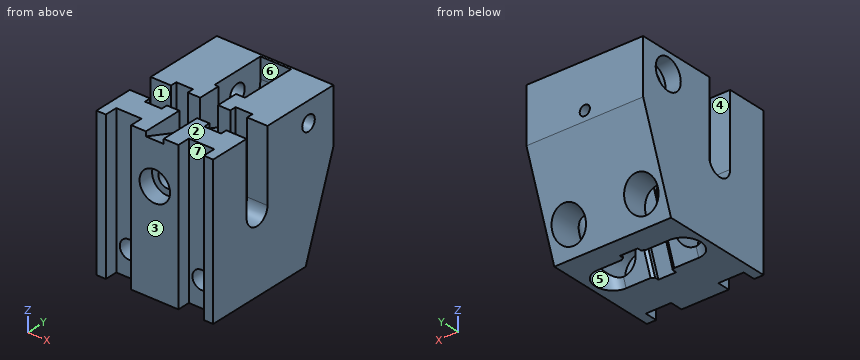
```python
from build123d import *

# Parameters (mm, degrees)
SKETCH1_W                = 23
SKETCH1_H                = 32.5
BOSS_EXTRUDE1_DEPTH      = 18
SKETCH2_W                = 23
SKETCH2_H                = 25
BOSS_EXTRUDE2_DEPTH      = 15
CHAMFER1_SIZE            = 15
SKETCH3_R                = 1.8
CUT_EXTRUDE1_DEPTH       = 44.694965385
CUT_EXTRUDE2_DEPTH       = 44.694965385
CUT_EXTRUDE3_START       = -4
CUT_EXTRUDE3_DEPTH       = 3.3
SKETCH7_W                = 5
SKETCH7_H                = 2.5
CUT_EXTRUDE4_DEPTH       = 52.713151132
CUT_EXTRUDE5_START       = -6.5
SKETCH8_R                = 3.25
CUT_EXTRUDE5_DEPTH       = 38.194965385
SKETCH9_R                = 1
CUT_EXTRUDE6_DEPTH       = 8
CUT_EXTRUDE8_DEPTH       = 1.75
CUT_EXTRUDE7_DEPTH       = 1.75
CUT_EXTRUDE9_DEPTH       = 13
SKETCH15_R               = 1.35
CUT_EXTRUDE10_DEPTH      = 6
CUT_EXTRUDE11_DEPTH      = 2.5
CUT_EXTRUDE11_DEPTH_BACK = 3.5
SKETCH17_R               = 1.75
CUT_EXTRUDE12_DEPTH      = 9
SKETCH18_R               = 3
CUT_EXTRUDE13_DEPTH      = 3
SKETCH19_R               = 1.5
CUT_EXTRUDE14_DEPTH      = 44.694965459
SKETCH20_R               = 1.75
CUT_EXTRUDE15_DEPTH      = 8
SKETCH21_R               = 3
CUT_EXTRUDE16_DEPTH      = 3
SKETCH22_R               = 1.5
CUT_EXTRUDE17_DEPTH      = 17
CUT_EXTRUDE18_DEPTH      = 44.694965459


with BuildPart() as part:
    # Sketch1 → Boss-Extrude1 (new body)
    with BuildSketch(Plane.XY):
        with Locations((11.5, 16.25)):
            Rectangle(SKETCH1_W, SKETCH1_H)
    extrude(amount=BOSS_EXTRUDE1_DEPTH)

    # Sketch2 → Boss-Extrude2 (add)
    with BuildSketch(Plane(origin=(0, 0, 0), x_dir=(-1, 0, 0), z_dir=(0, 0, -1))):
        with Locations((-11.5, 12.5)):
            Rectangle(SKETCH2_W, SKETCH2_H)
    extrude(amount=BOSS_EXTRUDE2_DEPTH)

    # Chamfer1
    # the kernel refuses this chamfer: 15 mm, written as the material it adds along each edge
    with BuildSketch(Plane(origin=(23, 25, 0), x_dir=(0, -0.02749587661058632, -0.9996219169112968), z_dir=(-1, 0, 0))) as chamfer1_piece_1_section:
        Polygon((CHAMFER1_SIZE * 0.999621916911, -CHAMFER1_SIZE * 0.0274958766106), (-CHAMFER1_SIZE * 0.0274958766106, -CHAMFER1_SIZE * 0.999621916911), (0, 0), align=None)
    chamfer1_piece_1 = extrude(amount=23, mode=Mode.PRIVATE)
    chamfer1_piece_1 = split(chamfer1_piece_1, bisect_by=Plane(origin=(11.5, 28.131672391, -15), z_dir=(0, 0, 1)), keep=Keep.TOP, mode=Mode.PRIVATE)
    chamfer1_piece_1 = split(chamfer1_piece_1, bisect_by=Plane(origin=(11.5, 32.5, -5.879790556), z_dir=(0, -1, 0)), keep=Keep.TOP, mode=Mode.PRIVATE)
    add(chamfer1_piece_1)

    # Sketch3 → Cut-Extrude1 (cut, through all)
    with BuildSketch(Plane.XZ):
        with Locations(Location((4.35, -10, 0), (0, 0, 270))):
            Circle(SKETCH3_R)
        with Locations(Location((18.65, -10, 0), (0, 0, 270))):
            Circle(SKETCH3_R)
    extrude(amount=-CUT_EXTRUDE1_DEPTH, mode=Mode.SUBTRACT)

    # Sketch4 → Cut-Extrude2 (cut, through all)
    with BuildSketch(Plane.ZY):
        with BuildLine():
            Line((0, 13), (18, 13))
            Line((18, 13), (18, 8))
            Line((18, 8), (0, 8))
            ThreePointArc((0, 8), (-2.5, 10.5), (0, 13))
        make_face()
    extrude(amount=-CUT_EXTRUDE2_DEPTH, mode=Mode.SUBTRACT)

    # Sketch5 → Cut-Extrude3 (cut)
    with BuildSketch(Plane.ZY.offset(CUT_EXTRUDE3_START)):
        Polygon((2.165063509, 14.25), (-2.165063509, 14.25), (-4.330127019, 10.5), (-2.165063509, 6.75), (2.165063509, 6.75), (18, 6.75), (18, 14.25), align=None)
    cut_extrude3 = extrude(amount=-CUT_EXTRUDE3_DEPTH, mode=Mode.SUBTRACT)

    # Sketch7 → Cut-Extrude4 (cut, through all)
    with BuildSketch(Plane(origin=(0, 0, -15), x_dir=(-1, 0, 0), z_dir=(0, 0, -1))):
        with Locations((-4.35, 1.25)):
            Rectangle(SKETCH7_W, SKETCH7_H)
    cut_extrude4 = extrude(amount=-CUT_EXTRUDE4_DEPTH, mode=Mode.SUBTRACT)

    # Sketch8 → Cut-Extrude5 (cut, through all)
    with BuildSketch(Plane.XZ.offset(CUT_EXTRUDE5_START)):
        with Locations(Location((4.35, -10, 0), (0, 0, 270))):
            Circle(SKETCH8_R)
    cut_extrude5 = extrude(amount=-CUT_EXTRUDE5_DEPTH, mode=Mode.SUBTRACT)

    # Mirror1: Cut-Extrude3, Cut-Extrude4, Cut-Extrude5 across plane
    add(cut_extrude3.mirror(Plane.ZY.offset(-11.5)), mode=Mode.SUBTRACT)
    add(cut_extrude4.mirror(Plane.ZY.offset(-11.5)), mode=Mode.SUBTRACT)
    add(cut_extrude5.mirror(Plane.ZY.offset(-11.5)), mode=Mode.SUBTRACT)

    # Sketch9 → Cut-Extrude6 (cut)
    with BuildSketch(Plane(origin=(0, 32.5, 0), x_dir=(1, 0, 0), z_dir=(0, 1, 0))):
        with Locations(Location((11.5, -5.25, 0), (0, 0, 270))):
            Circle(SKETCH9_R)
    extrude(amount=-CUT_EXTRUDE6_DEPTH, mode=Mode.SUBTRACT)

    # Sketch10 → Cut-Extrude8 (cut, symmetric)
    with BuildSketch(Plane.ZY.offset(-11.5)):
        Polygon((4.25, 24.5), (18, -13.277814518), (31.330171166, -4.978014809), (56.797179747, 10.878576059), (6.25, 24.5), align=None)
    extrude(amount=CUT_EXTRUDE8_DEPTH, both=True, mode=Mode.SUBTRACT)

    # Sketch11 → Cut-Extrude7 (cut, symmetric)
    with BuildSketch(Plane.ZY.offset(-11.5)):
        Polygon((1.029605681, 24.137976813), (5.29394834, 23.386058148), (6.774939004, 19.317069741), (3.991587008, 16), (-15, 9.087627628), (-15, 18.303677479), align=None)
    extrude(amount=CUT_EXTRUDE7_DEPTH, both=True, mode=Mode.SUBTRACT)

    # Sketch12 → Cut-Revolve2 (revolve, cut)
    with BuildSketch(Plane.ZY.offset(-11.5)):
        Polygon((0.20282315, 23.485738747), (1.570903724, 19.726968263), (-16.480990664, 13.156616034), (-17.849071237, 16.915386518), align=None)
    revolve(axis=Axis((11.5, 19.726968263, 1.570903724), (0, -0.34202014332567215, -0.9396926207859072)), mode=Mode.SUBTRACT)

    # Sketch13 → Cut-Extrude9 (cut)
    with BuildSketch(Plane(origin=(0, -3.757856581, -10.324626103), x_dir=(1, 0, 0), z_dir=(0, 0.34202014332567177, 0.9396926207859073))):
        with BuildLine():
            Line((18.65, 21.250005791), (11.5, 21.250005791))
            Line((11.5, 21.250005791), (11.5, 14.750005791))
            Line((11.5, 14.750005791), (18.65, 14.750005791))
            ThreePointArc((18.65, 14.750005791), (21.9, 18.000005791), (18.65, 21.250005791))
        make_face()
    cut_extrude9 = extrude(amount=CUT_EXTRUDE9_DEPTH, mode=Mode.SUBTRACT)

    # Sketch15 → Cut-Extrude10 (cut)
    with BuildSketch(Plane(origin=(0, 0.688405282, 1.891377967), x_dir=(-1, 0, 0), z_dir=(0, -0.34202014332567177, -0.9396926207859073))):
        with Locations(Location((-18.65, 18.000005791, 0), (0, 0, 90))):
            Circle(SKETCH15_R)
    cut_extrude10 = extrude(amount=-CUT_EXTRUDE10_DEPTH, mode=Mode.SUBTRACT)

    # Mirror2: Cut-Extrude9, Cut-Extrude10 across plane
    add(cut_extrude9.mirror(Plane.ZY.offset(-11.5)), mode=Mode.SUBTRACT)
    add(cut_extrude10.mirror(Plane.ZY.offset(-11.5)), mode=Mode.SUBTRACT)

    # Sketch16 → Cut-Extrude11 (cut, two sides: drawn at the far end of the back side and taken through both)
    with BuildSketch(Plane.ZY.offset(-11.5).offset(-CUT_EXTRUDE11_DEPTH_BACK)):
        with BuildLine():
            Line((10.075121942, 28.322250561), (25.575121942, 28.322250561))
            Line((25.575121942, 28.322250561), (25.575121942, 17.322250561))
            Line((25.575121942, 17.322250561), (10.075121942, 17.322250561))
            ThreePointArc((10.075121942, 17.322250561), (4.575121942, 22.822250561), (10.075121942, 28.322250561))
        make_face()
    extrude(amount=CUT_EXTRUDE11_DEPTH + CUT_EXTRUDE11_DEPTH_BACK, mode=Mode.SUBTRACT)

    # Sketch17 → Cut-Extrude12 (cut)
    with BuildSketch(Plane.ZY):
        with Locations((10.075121942, 22.822250561)):
            Circle(SKETCH17_R)
    extrude(amount=-CUT_EXTRUDE12_DEPTH, mode=Mode.SUBTRACT)

    # Sketch18 → Cut-Extrude13 (cut)
    with BuildSketch(Plane.ZY):
        with Locations((10.075121942, 22.822250561)):
            Circle(SKETCH18_R)
    extrude(amount=-CUT_EXTRUDE13_DEPTH, mode=Mode.SUBTRACT)

    # Sketch19 → Cut-Extrude14 (cut, through all)
    with BuildSketch(Plane.ZY):
        with Locations((10.075121942, 22.822250561)):
            Circle(SKETCH19_R)
    extrude(amount=-CUT_EXTRUDE14_DEPTH, mode=Mode.SUBTRACT)

    # Sketch20 → Cut-Extrude15 (cut)
    with BuildSketch(Plane.XZ):
        with Locations(Location((11.5, 5, 0), (0, 0, 270))):
            Circle(SKETCH20_R)
    extrude(amount=-CUT_EXTRUDE15_DEPTH, mode=Mode.SUBTRACT)

    # Sketch21 → Cut-Extrude16 (cut)
    with BuildSketch(Plane.XZ):
        with Locations(Location((11.5, 5, 0), (0, 0, 270))):
            Circle(SKETCH21_R)
    extrude(amount=-CUT_EXTRUDE16_DEPTH, mode=Mode.SUBTRACT)

    # Sketch22 → Cut-Extrude17 (cut)
    with BuildSketch(Plane.XZ):
        with Locations(Location((11.5, 5, 0), (0, 0, 222.242919533))):
            Circle(SKETCH22_R)
    extrude(amount=-CUT_EXTRUDE17_DEPTH, mode=Mode.SUBTRACT)

    # Sketch23 → Cut-Extrude18 (cut, through all)
    with BuildSketch(Plane(origin=(0, 0, 0), x_dir=(0, 0, -1), z_dir=(1, 0, 0))):
        Polygon((-18, 32.5), (-14.075121942, 32.5), (-13.4247686, 32.5), (15, 32.5), (15, 22.154230314), (-3.320235061, 28.822250561), (-14.075121942, 28.822250561), (-14.075121942, 0), (-18, 0), align=None)
    extrude(amount=CUT_EXTRUDE18_DEPTH, mode=Mode.SUBTRACT)


solid = part.part
```
The model under review builds one solid part; all positions refer to its coordinate system, in mm. Face numbers are marked on the shaded views. A direction names the side the tool comes from. Round coordinates to 2 decimals unless told otherwise and drop trailing zeros. Loops run counter-clockwise (first coordinate to the right, second up) from the corner with the lowest first, then second, coordinate; pieces in that order, holes last. Notation, with made-up numbers: M 5,70.5 L 53,70.5 A22 cw 53,106.5 Z; hole C 62,58.25 d7. An arc over 180 degrees is marked long. Put each result on its own line as item: value.
Q1. Machinability: for the marked faces 4, 5, 6 and 7, which of the approach directions +Z, -Z, +X, -X, +Y, -Y give a long, thin tool a straight path to every point of the face, cutting with its end or side? Answer none if there is none.
Result set:
face 4: +Z, +X, -X
face 5: none
face 6: +Z
face 7: +Z, -Z, -Y
Q2. Consider section A-A, the plane y = 8.5. Give the boundary of the cut face in (x, z).
Result set:
outline: M 0,-15 L 23,-15 L 23,-1.5 L 19,-1.5 L 19,-3.18 L 15.7,-3.18 L 15.7,-1.5 L 7.3,-1.5 L 7.3,-3.18 L 4,-3.18 L 4,-1.5 L 0,-1.5 Z; hole C 4.35,-10 d6.5; hole C 18.65,-10 d6.5
Q3. To check wall thickness, follow L1, parallel to X at y = 7.05, z = 5; L2, parallel to X at y = 19.25, z = 11.5; L3, parallel to X at y = 16, z = 5. State the ranges of each line that lie inside material, in increasing order.
Result set:
L1: x = 0 to 4, 7.3 to 9.75, 13.25 to 15.7, 19 to 23
L2: x = 0 to 9, 15 to 23
L3: x = 0 to 10, 13 to 23
Q4. For pin 1 (5 mm diameter, centred on y = 19.5, z = 0.5, fed in from -X); pin 2 (12 mm diameter, centred on x = 6.5, z = -6.5, fed in from +Y); pin 3 (1.2 mm diameter, centred on x = 11.5, z = 5.25, fed in from +Y); pin 4 (1.8 mm diameter, centred on x = 10.5, z = 4, fed in from -Y), all flat-tipped, find the tip position at first contact; note any pin that passes through.
Result set:
pin 1: stops at x = 0
pin 2: stops at y = 27.43
pin 3: stops at y = 18.21
pin 4: stops at y = 3
Q5. Mouldability with a two-part tool opening along Y and no side actions: class the marked faces 1, 2 and 3 as released by +Y, released by -Y, zero draft, split by the parting line, or undercut.
Result set:
face 1: undercut
face 2: zero draft
face 3: released by -Y
Q6. Consider section C-C, the plane z = 5.25. Count the separate pieces of the cut face and the enclosed holes in it, then the cut area to 3 significant figures.
Result set:
separate pieces: 3
enclosed holes: 0
area: 412 mm²
Q7. Consider section B-B, the plane x = 8. Give the boundary of the cut face in (y, z), then the cut area to 3 significant figures.
Result set:
outline: M 0,-15 L 10.24,-15 L 14.55,-3.15 L 15.78,-3.6 L 17.91,2.23 L 21.55,0.91 L 19.42,-4.93 L 20.66,-5.38 L 17.15,-15 L 22.15,-15 L 28.82,3.32 L 28.82,14.08 L 13,14.08 L 13,0 A2.5 cw 8,0 L 8,14.08 L 0,14.08 Z; hole C 22.82,10.08 d3.5
area: 589 mm²
